The model under review builds one solid part; all positions refer to its coordinate system, in mm. A direction names the side the tool comes from. Round coordinates to 2 decimals unless told otherwise and drop trailing zeros. Order: outer loops, then holes, each group sorted by start corner. A loop starts at its lowest first (then second) coordinate and runs counter-clockwise, first axis right, second up.
1) Consider section C-C (z = -6). Give the boundary of the cut face in (x, y), then the cut area to 3 significant figures.
2) Consider section A-A (x = 13). Give the number of separate pieces and of enclosed holes in the cut face, then the cut area to 3 significant figures.
3) Machinability: for faces 1 (the face through (15.177, 2.958, -10.078)), 2 (the face through (13, 5, -4.679)), 3 (the face through (12, 7.8, -10)), which of the approach directions +Z, -Z, +X, -X, +Y, -Y give a long, thin tool a straight path to every point of the face, cutting with its end or side? Answer none if there is none.
4) Consider section B-B (y = 7). Give the boundary of the cut face in (x, z), then the cut area to 3 significant figures.
5) To check wall thickness, follow L1, parallel to Z at x = 10, y = 8.75; L2, parallel to Z at x = 11.75, y = 15.25; L3, parallel to X at y = 8.5, z = -1.25. State the ranges of each line that lie inside material, in increasing order.
6) Clearance check with flat-ended pins moving along their axes: P1, Ø1.2, axis at x = 2.5, z = -2.5, coming from the +Y side; P2, Ø1.2, axis at x = 13, z = -10.5, coming from the +Y side; P3, Ø1.5, axis at x = 13, z = -6, coming from the -Y side; P4, Ø1.5, axis at y = 4.5, z = -6.5, coming from the -X side. State where each tip first meets the part, or that it passes through.
7) Mouldability with a two-part tool opening along X and no side actions: class faces 4 (the face through (1.37, 10.14, -14.11)), 5 (the face through (9.77, 5, -6)), 6 (the face through (12, 6, -10)) as pulls with the +X half, pulls with the -X half, needs draft (parallel to the pull), parting line crosses it, or undercut.
8) Consider section D-D (x = 5). Give the boundary of the cut face in (y, z), then the cut area to 3 significant figures.
Autodesk Fusion 360 part; units mm, degrees
sketch "Sketch1" plane through (0, 0, 0) normal (0, 1, 0) x (1, 0, 0)
  line L0 (0.7695, -2.3211) -> (15.7695, -2.3211)
  line L1 (15.7695, -2.3211) -> (15.7695, 4.6789)
  line L2 (0.7695, 4.6789) -> (0.7695, -2.3211)
  line L3 (15.7695, 7.6789) -> (15.7695, 14.6789)
  line L4 (0.7695, 14.6789) -> (0.7695, 7.6789)
  line L5 (15.7695, 14.6789) -> (0.7695, 14.6789)
  line L6 (9.7695, 4.6789) -> (9.7695, 7.6789)
  line L7 (8.7695, 7.6789) -> (8.7695, 4.6789)
  circle A0 centre (8.2695, 1.6789) radius 2
  line L8 (15.7695, 4.6789) -> (9.7695, 4.6789)
  line L9 (8.7695, 4.6789) -> (0.7695, 4.6789)
  line L10 (0.7695, 7.6789) -> (8.7695, 7.6789)
  line L11 (9.7695, 7.6789) -> (15.7695, 7.6789)
  circle A1 centre (13.2695, 1.6789) radius 2
  circle A2 centre (3.2695, 1.6789) radius 2
  circle A3 centre (8.2695, 10.6789) radius 2
  circle A4 centre (13.2695, 10.6789) radius 2
  circle A5 centre (3.2695, 10.6789) radius 2
  circle A6 centre (-6.7305, 1.6789) radius 1
  circle A7 centre (-11.7305, 1.6789) radius 1
  circle A8 centre (-16.7305, 1.6789) radius 1
  line L12 (-4.7305, -1.3211) -> (-18.7305, -1.3211)
  line L13 (-18.7305, -1.3211) -> (-18.7305, 3.6789)
  line L14 (-18.7305, 3.6789) -> (-4.7305, 3.6789)
  line L15 (-4.7305, 3.6789) -> (-4.7305, -1.3211)
  circle A9 centre (-6.7305, 10.6789) radius 1
  circle A10 centre (-16.7305, 10.6789) radius 1
  circle A11 centre (-11.7305, 10.6789) radius 1
  line L16 (-4.7305, 8.6789) -> (-18.7305, 8.6789)
  line L17 (-4.7305, 13.6789) -> (-4.7305, 8.6789)
  line L18 (-18.7305, 13.6789) -> (-4.7305, 13.6789)
  line L19 (-18.7305, 8.6789) -> (-18.7305, 13.6789)
  line L20 (20.7695, 3.6789) -> (35.7695, 3.6789)
  line L21 (35.7695, 3.6789) -> (35.7695, 8.6789)
  line L22 (35.7695, 8.6789) -> (20.7695, 8.6789)
  line L23 (20.7695, 8.6789) -> (20.7695, 3.6789)
  dimension "d1" = 15
  dimension "d2" = 7
  dimension "d3" = 15
  dimension "d4" = 7
  dimension "d6" = 6
  dimension "d7" = 4
  dimension "d8" = 4
  dimension "d9" = 4
  dimension "d10" = 5
  dimension "d11" = 5
  dimension "d12" = 4
  dimension "d13" = 2.5
  dimension "d14" = 4
  dimension "d15" = 4
  dimension "d16" = 4
  dimension "d17" = 5
  dimension "d18" = 5
  dimension "d21" = 2
  dimension "d22" = 2
  dimension "d23" = 2
  dimension "d24" = 14
  dimension "d25" = 5
  dimension "d27" = 1
  dimension "d29" = 5
  dimension "d30" = 5
  dimension "d31" = 3
  dimension "d32" = 20.5
  dimension "d33" = 2
  dimension "d34" = 2
  dimension "d35" = 2
  dimension "d36" = 2
  dimension "d37" = 14
  dimension "d38" = 5
  dimension "d39" = 5
  dimension "d40" = 5
  dimension "d41" = 2
  dimension "d42" = 2
  dimension "d43" = 1
  dimension "d49" = 5
  dimension "d50" = 15
  dimension "d51" = 20
extrude "Extrude4" add sketch "Sketch1" along normal blind 20 contours L0 L1 L2 L3 L4 L5 L6 L7 L8 L9 L10 L11 makes body 1
extrude "Extrude5" add sketch "Sketch1" along normal blind 1.8 separate body contours L12 L13 L14 L15 | L16 L17 L18 L19 makes body 2 at (-11.7056, 0, 0.6535) makes body 3 at (-11.7555, 0, -13.0113)
move_body "Move2" bodies 2 3 to x (1, 0, 0) y (0, 1, 0) z (0, 0, 1) at (20, 6, 0)
extrude "Extrude6" add sketch "Sketch1" along normal blind 10 separate body contours L20 L21 L22 L23 makes body 4
move_body "Move4" bodies 4 to x (1, 0, 0) y (0, 1, 0) z (0, 0, 1) at (0, 10, 0)
move_body "Move5" bodies 4 to x (1, 0, 0) y (0, 1, 0) z (0, 0, 1) at (-20, 0, 0)
combine "Combine1" operation add target body 1 tool bodies 3 4 2
fillet "Fillet5" radius 2 1 edges at (15.7695, 10, -14.6789) on bodies 1
fillet "Fillet6" radius 2 1 edges at (0.7695, 10, -14.6789) on bodies 1
fillet "Fillet7" radius 2 1 edges at (0.7695, 10, 2.3211) on bodies 1
fillet "Fillet8" radius 2 1 edges at (15.7695, 10, 2.3211) on bodies 1
Answer below:
1. outline: (0.77, 10) - (8.77, 10) - (8.77, 0) - (9.77, 0) - (9.77, 10) - (15.77, 10) - (15.77, 20) - (0.77, 20) - close
1. area: 160 mm2
2. separate pieces: 3
2. enclosed holes: 0
2. area: 159 mm2
3. face 1: -Y
3. face 2: +X, -Y
3. face 3: +Y
4. outline: (0.77, -12.68) arc R2 ccw to (2.77, -14.68) - (13.77, -14.68) arc R2 ccw to (15.77, -12.68) - (15.77, -7.68) - (9.77, -7.68) - (9.77, -4.68) - (15.77, -4.68) - (15.77, 0.32) arc R2 ccw to (13.77, 2.32) - (2.77, 2.32) arc R2 ccw to (0.77, 0.32) - (0.77, -4.68) - (8.77, -4.68) - (8.77, -7.68) - (0.77, -7.68) - close; hole circle Ø2 at (3.27, -10.68); hole circle Ø2 at (3.27, -1.68); hole circle Ø2 at (8.27, -10.68); hole circle Ø2 at (8.27, -1.68); hole circle Ø2 at (13.27, -10.68); hole circle Ø2 at (13.27, -1.68)
4. area: 191 mm2
5. L1: z = -14.68 to -11.68, -9.68 to -7.68, -4.68 to -2.68, -0.68 to 2.32
5. L2: z = -14.68 to -11.98, -9.38 to -2.98, -0.38 to 2.32
5. L3: x = 0.77 to 1.32, 5.22 to 6.32, 10.22 to 11.32, 15.22 to 15.77
6. P1: stops at y = 7.8
6. P2: passes through
6. P3: stops at y = 10
6. P4: stops at x = 8.77
7. face 4: pulls with the -X half
7. face 5: pulls with the +X half
7. face 6: undercut
8. outline: (0, -14.68) - (20, -14.68) - (20, -11.68) - (7.8, -11.68) - (7.8, -9.68) - (20, -9.68) - (20, -2.68) - (7.8, -2.68) - (7.8, -0.68) - (20, -0.68) - (20, 2.32) - (0, 2.32) - (0, -0.68) - (6, -0.68) - (6, -2.68) - (0, -2.68) - (0, -4.68) - (10, -4.68) - (10, -7.68) - (0, -7.68) - (0, -9.68) - (6, -9.68) - (6, -11.68) - (0, -11.68) - close
8. area: 237 mm2
